Here's the drawing with two shaded views (mm, measured from the low corner). I have some questions. A direction names the side the tool comes from. Round coordinates to 2 decimals unless told otherwise and drop trailing zeros. Loops run counter-clockwise (first coordinate to the right, second up) from the corner with the lowest first, then second, coordinate; pieces in that order, holes last. Notation, with made-up numbers: (29.5, 51.5) -> (57.5, 51.5) arc R19 ccw to (57.5, 82.5) -> close; hole circle Ø2 at (-20.75, 5). An arc over 180 degrees is marked (long way). One line per item, written item: value. Start each with the question number.
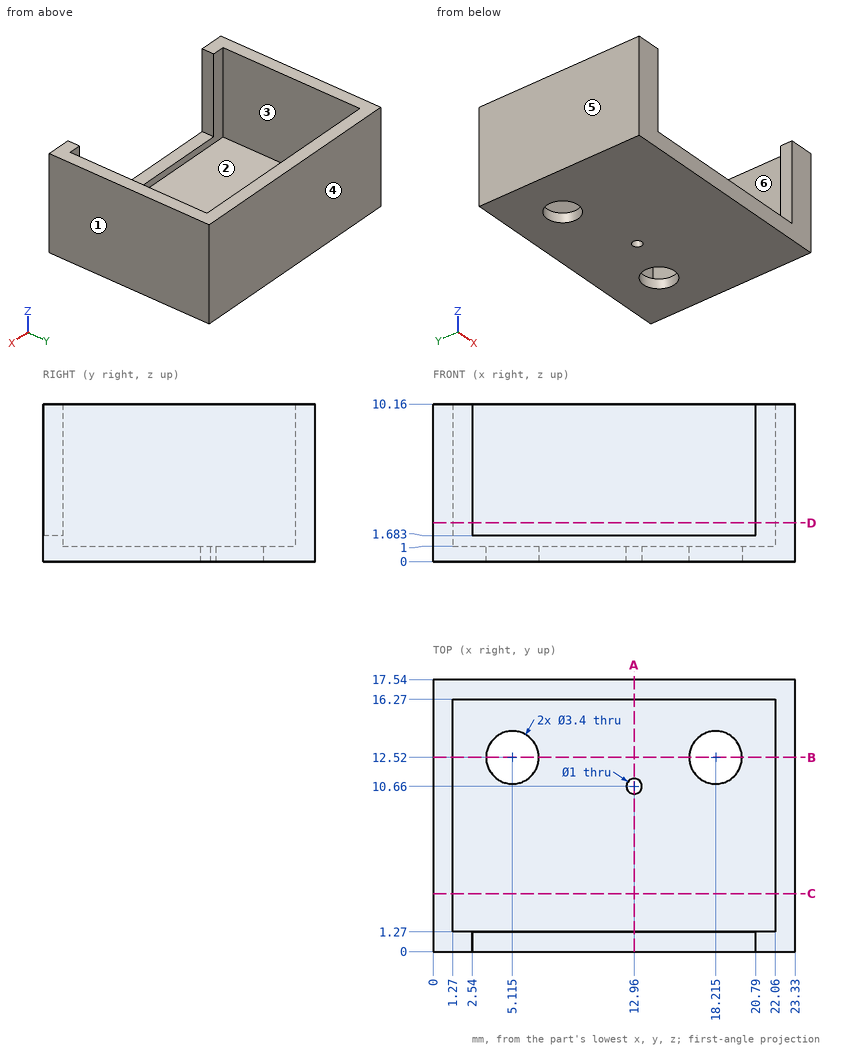
Q1. If I drill on line 1 along X through (y, z) = (11.5, 7); line 2 along X through (y, z) = (1, 3.25); line 3 along Y through (x, z) = (2.75, 1.5), over which ranges is the centre line in solid material (lowest first)?
Q2. I want a section at B-B on y = 12.52. Please give me the cut outline in (x, z) (1 decimal), plus the area to 3 significant figures.
Q3. Which directions (+Z, -Z, +X, -X, +Y, -Y) give clear straight access to the entire face, cutting with the end or side of a thin tool? Please do the marked faces 5 and 6.
Q4. I want a section at A-A on x = 12.96. Please give me the cut outline in (y, z).
Q5. Will these pins go through, and if not, where does the flat tip stop? P1, Ø1, axis at x = 9, y = 0.5, coming from the +Z side; P2, Ø5.5, axis at x = 18.215, y = 12.52, coming from the +Z side; P3, Ø4, axis at y = 6.5, z = 5, coming from the -X side; P4, Ø2.5, axis at x = 5.115, y = 12.52, coming from the +Z side.
Q6. I want a section at C-C on y = 3.75. Please give me the cut outline in (x, z).
Q7. If we mould it in two halves opening along Y, with no side actions, what happens to the marked faces 1, 2, 3 and 4? For each: released by +Y, released by -Y, zero draft, split by the parting line, or undercut.
Q8. I want a section at D-D on z = 2.5. Please give me the cut outline in (x, y).
Answers below:
1. line 1: x = 0 to 1.27, 22.06 to 23.33
1. line 2: x = 0 to 2.54, 20.79 to 23.33
1. line 3: y = 0 to 1.27, 16.27 to 17.54
2. outline: (0, 0) -> (3.4, 0) -> (3.4, 1) -> (1.3, 1) -> (1.3, 10.2) -> (0, 10.2) -> close; (6.8, 0) -> (16.5, 0) -> (16.5, 1) -> (6.8, 1) -> close; (19.9, 0) -> (23.3, 0) -> (23.3, 10.2) -> (22.1, 10.2) -> (22.1, 1) -> (19.9, 1) -> close
2. area: 39.8 mm^2
3. face 5: +Z, -Z, -X, +Y, -Y
3. face 6: +Z
4. outline: (0, 0) -> (10.16, 0) -> (10.16, 1) -> (1.27, 1) -> (1.27, 1.68) -> (0, 1.68) -> close; (11.16, 0) -> (17.54, 0) -> (17.54, 10.16) -> (16.27, 10.16) -> (16.27, 1) -> (11.16, 1) -> close
5. P1: stops at z = 1.68
5. P2: stops at z = 1
5. P3: stops at x = 0
5. P4: passes through
6. outline: (0, 0) -> (23.33, 0) -> (23.33, 10.16) -> (22.06, 10.16) -> (22.06, 1) -> (1.27, 1) -> (1.27, 10.16) -> (0, 10.16) -> close
7. face 1: zero draft
7. face 2: undercut
7. face 3: undercut
7. face 4: released by +Y
8. outline: (0, 0) -> (2.54, 0) -> (2.54, 1.27) -> (1.27, 1.27) -> (1.27, 16.27) -> (22.06, 16.27) -> (22.06, 1.27) -> (20.79, 1.27) -> (20.79, 0) -> (23.33, 0) -> (23.33, 17.54) -> (0, 17.54) -> close
